The listing builds one solid part. Answer for the finished solid, in the listing's coordinates (mm). A direction names the side the tool comes from. Round coordinates to 2 decimals unless told otherwise and drop trailing zeros. Write each loop counter-clockwise with the first axis right and the second up, starting at its lowest first coordinate (ties: lowest second). Pieces come first, ordered by that corner, then holes. Notation, with made-up numbers: M 43,64.5 L 91,64.5 A10 cw 91,79.5 Z; hole C 36,30 d3. An arc over 180 degrees is marked long. One line per item, written item: value. Start each with the question number.
(1) For faces 1 (the cylindrical face through (9.9, 15.5, 1.5)), 2 (the cylindrical face through (-4.906, 14.429, 1.503)), 3 (the flat face through (12.941, -2, 2)), determine the directions among +Z, -Z, +X, -X, +Y, -Y from which every point of the face is accessible in a straight line to the end or side of a thin tool.
(2) Section B-B (x = 6) is taken. Determine the outline of the cut face in (y, z).
(3) For a pull along Y with two mould halves and no side action, classify faces 4 (the flat face through (5, -8.915, 2)), 5 (the cylindrical face through (-12.466, -12.79, 1.545)), 6 (the flat face through (-8, -8, 3.048)) as released by +Y, released by -Y, zero draft, split by the parting line, or undercut.
(4) Consider probe 1 along Y at (x, z) = (12, 1.6); probe 2 along Y at (x, z) = (13.5, 0.7); probe 3 along Y at (x, z) = (-2.5, 2.65). Determine where each line is inside the solid, lowest interval first.
(5) Section D-D (z = 0.9) is taken. State how many separate pieces and enclosed holes the cut face has, plus the area to 3 significant figures.
(6) Given P1, Ø1.5, axis at y = -6.5, z = 2, coming from the -X side; P2, Ø0.5, axis at y = -8.5, z = 1.5, coming from the +X side; P3, Ø0.8, axis at x = -15.5, z = 1, coming from the -Y side; P4, Ø5, axis at x = -11, y = -7.5, coming from the -Z side, each flat-ended and moving along its own axis, determine where each tip first touches the part or whether it passes through.
(7) Section A-A (x = 0) is taken. Determine the outline of the cut face in (y, z).
(8) Section C-C (y = 0.5) is taken. Determine the outline of the cut face in (x, z), plus the area to 3 significant figures.
```python
from build123d import *

# Parameters (mm, degrees)
SKETCH1_R           = 1.4224
BOSS_EXTRUDE1_DEPTH = 3.048
CUT_EXTRUDE1_DEPTH  = 31.684629768
SKETCH3_R           = 21.59
SKETCH3_R_2         = 17.859965052
CUT_EXTRUDE2_DEPTH  = 31.684629768
SKETCH4_R           = 1.524
SKETCH4_R_2         = 1.8415
BOSS_EXTRUDE3_DEPTH = 3.048
SKETCH7_W           = 0.508
SKETCH7_H           = 3.683
BOSS_EXTRUDE4_DEPTH = 3.048


with BuildPart() as part:
    # Sketch1 → Boss-Extrude1 (new body)
    with BuildSketch(Plane.XY):
        with BuildLine():
            Line((-14.952058744, -2.948480848), (-16.984058744, -2.948480848))
            Line((-16.984058744, -2.948480848), (-16.984058744, -5.5245))
            Line((-16.984058744, -5.5245), (-20.871224203, -5.5245))
            ThreePointArc((-20.871224203, -5.5245), (21.59, 0), (-20.871224203, 5.5245))
            Line((-20.871224203, 5.5245), (-16.984058744, 5.5245))
            Line((-16.984058744, 5.5245), (-16.984058744, 2.948480848))
            Line((-16.984058744, 2.948480848), (-14.952058744, 2.948480848))
            ThreePointArc((-14.952058744, 2.948480848), (-13.968818521, 6.093415226), (-12.332576282, 8.9535))
            Line((-12.332576282, 8.9535), (-7.9248, 7.366))
            Line((-7.9248, 7.366), (-7.9248, 3.302))
            Line((-7.9248, 3.302), (-5.6007, 3.302))
            Line((-5.6007, 3.302), (-5.6007, 14.173558463))
            ThreePointArc((-5.6007, 14.173558463), (-4.895856129, 14.43219293), (-4.179129857, 14.6558))
            Line((-4.179129857, 14.6558), (4.179129857, 14.6558))
            Line((4.179129857, 14.6558), (11.43, 14.6558))
            Line((11.43, 14.6558), (11.43, -0.8128))
            Line((11.43, -0.8128), (12.9413, -0.8128))
            Line((12.9413, -0.8128), (12.9413, -4.064))
            Line((12.9413, -4.064), (8.4582, -4.064))
            Line((8.4582, -4.064), (8.4582, -8.9154))
            Line((8.4582, -8.9154), (1.2573, -8.9154))
            Line((1.2573, -8.9154), (1.2573, -7.3406))
            Line((1.2573, -7.3406), (-0.7747, -8.8265))
            Line((-0.7747, -8.8265), (-3.273729572, -11.3919))
            Line((-3.273729572, -11.3919), (-5.093162196, -9.619538602))
            Line((-5.093162196, -9.619538602), (-4.769706241, -9.287492148))
            Line((-4.769706241, -9.287492148), (-9.167166743, -5.0038))
            Line((-9.167166743, -5.0038), (-14.395123673, -5.0038))
            ThreePointArc((-14.395123673, -5.0038), (-14.709533071, -3.985879682), (-14.952058744, -2.948480848))
        make_face()
        with Locations(Location((0, 18.415, 0), (0, 0, 180))):
            Circle(SKETCH1_R, mode=Mode.SUBTRACT)
        with Locations(Location((0, -18.415, 0), (0, 0, 180))):
            Circle(SKETCH1_R, mode=Mode.SUBTRACT)
    extrude(amount=BOSS_EXTRUDE1_DEPTH)

    # Sketch2 → Cut-Extrude1 (cut, through all)
    with BuildSketch(Plane.XY.offset(3.048)):
        Polygon((-14.395123673, -5.0038), (-16.984058744, -5.5245), (-16.984058744, 5.5245), (-14.203432675, 5.5245), align=None)
    extrude(amount=-CUT_EXTRUDE1_DEPTH, mode=Mode.SUBTRACT)

    # Sketch3 → Cut-Extrude2 (cut, through all)
    with BuildSketch(Plane.XY.offset(3.048)):
        Circle(SKETCH3_R)
        Circle(SKETCH3_R_2, mode=Mode.SUBTRACT)
    extrude(amount=-CUT_EXTRUDE2_DEPTH, mode=Mode.SUBTRACT)


with BuildPart() as cut_extrude2_piece_1:
    # of the separate pieces the step leaves, piece 1, a body of its own (cut_extrude2_pieces)
    add(part.part.solids().sort_by_distance((-14.395123673, -5.0038, 0))[0])



with BuildPart() as cut_extrude2_piece_2:
    # of the separate pieces the step leaves, piece 2, a body of its own (cut_extrude2_pieces)
    add(part.part.solids().sort_by_distance((-16.984058744, 5.5245, 0))[0])


with BuildPart() as cut_extrude2_piece_1_1:
    add(cut_extrude2_piece_1.part)

    add(cut_extrude2_piece_2.part)  # Boss-Extrude3 merges Cut-Extrude2 piece 2
    # Sketch4 → Boss-Extrude3 (add)
    # profile 1 of 4: a face of its own
    with BuildSketch(Plane.XY.offset(3.048)):
        with BuildLine():
            ThreePointArc((8.770915547, 15.557936629), (9.49974685, 15.123926787), (10.207148379, 14.6558))
            Line((10.207148379, 14.6558), (11.43, 14.6558))
            Line((11.43, 14.6558), (11.43, 13.723463545))
            ThreePointArc((11.43, 13.723463545), (12.531489365, 12.72556977), (13.546192441, 11.639545611))
            ThreePointArc((13.546192441, 11.639545611), (13.259158271, 12.690113644), (13.891550536, 13.576771317))
            ThreePointArc((13.891550536, 13.576771317), (14.229434963, 17.341171724), (10.603438482, 16.274857592))
            ThreePointArc((10.603438482, 16.274857592), (9.857305907, 15.481530348), (8.770915547, 15.557936629))
        make_face()
        with Locations((12.779339593, 15.573965052)):
            Circle(SKETCH4_R, mode=Mode.SUBTRACT)
    # profile 2 of 4: a face of its own
    with BuildSketch(Plane.XY.offset(3.048)):
        with BuildLine():
            ThreePointArc((-1.288911844, 17.813395463), (0, 16.9926), (1.288911844, 17.813395463))
            ThreePointArc((1.288911844, 17.813395463), (0, 17.859965052), (-1.288911844, 17.813395463))
        make_face()
    # profile 3 of 4: a face of its own
    with BuildSketch(Plane.XY.offset(3.048)):
        with BuildLine():
            ThreePointArc((-8.770915605, 15.557936596), (-9.857305878, 15.481530337), (-10.603438442, 16.274857469))
            ThreePointArc((-10.603438442, 16.274857469), (-14.229434898, 17.341171777), (-13.891550571, 13.576771336))
            ThreePointArc((-13.891550571, 13.576771336), (-13.259158271, 12.690113644), (-13.546192467, 11.639545581))
            ThreePointArc((-13.546192467, 11.639545581), (-11.329244247, 13.806758362), (-8.770915605, 15.557936596))
        make_face()
        with Locations((-12.779339593, 15.573965052)):
            Circle(SKETCH4_R, mode=Mode.SUBTRACT)
    # profile 4 of 4: a face of its own
    with BuildSketch(Plane.XY.offset(3.048)):
        with BuildLine():
            ThreePointArc((3.078011458, -20.256202915), (3.341190672, -18.362372873), (4.85058289, -17.188664791))
            ThreePointArc((4.85058289, -17.188664791), (3.085598969, -17.591402181), (1.288911844, -17.813395463))
            ThreePointArc((1.288911844, -17.813395463), (0, -16.9926), (-1.288911844, -17.813395463))
            ThreePointArc((-1.288911844, -17.813395463), (-3.085599014, -17.591402173), (-4.850582978, -17.188664766))
            ThreePointArc((-4.850582978, -17.188664766), (-3.341190697, -18.36237283), (-3.078011456, -20.256202907))
            ThreePointArc((-3.078011456, -20.256202907), (-4e-09, -24.209965052), (3.078011458, -20.256202915))
        make_face()
        with Locations((0, -21.034965052)):
            Circle(SKETCH4_R_2, mode=Mode.SUBTRACT)
    extrude(amount=-BOSS_EXTRUDE3_DEPTH)

    # Sketch7 → Boss-Extrude4 (add)
    with BuildSketch(Plane.XY.offset(3.048)):
        with Locations((11.176, 12.8143)):
            Rectangle(SKETCH7_W, SKETCH7_H)
    extrude(amount=-BOSS_EXTRUDE4_DEPTH)


solid = cut_extrude2_piece_1_1.part
```
Recorded:
1. face 1: +Z, -Z, +Y
1. face 2: +Z, -Z
1. face 3: +Z, -Z, -X
2. outline: M -16.82,0 L -8.92,0 L -8.92,3.05 L -16.82,3.05 Z; M 14.66,0 L 16.82,0 L 16.82,3.05 L 14.66,3.05 Z
3. face 4: undercut
3. face 5: released by -Y
3. face 6: zero draft
4. probe 1: y = -13.23 to -4.06, -0.81 to 14.26, 16.88 to 17.72
4. probe 2: y = -11.69 to 11.7, 13.24 to 14.23, 16.92 to 17.74
4. probe 3: y = -22.99 to -10.6, 14.66 to 17.68
5. separate pieces: 1
5. enclosed holes: 3
5. area: 514 mm2
6. P1: stops at x = -16.91
6. P2: stops at x = 15.84
6. P3: stops at y = -9.54
6. P4: stops at z = 0
7. outline: M -24.21,0 L -22.88,0 L -22.88,3.05 L -24.21,3.05 Z; M -19.19,0 L -8.26,0 L -8.26,3.05 L -19.19,3.05 Z; M 14.66,0 L 17.86,0 L 17.86,3.05 L 14.66,3.05 Z
8. outline: M 11.43,0 L 17.85,0 L 17.85,3.05 L 11.43,3.05 Z
8. area: 19.6 mm2
